Verification items for this drawing (mm, ordinates from the low corner). Coordinates: 2 decimals unless noted, no trailing zeros. Write each loop counter-clockwise with the first axis right and the second up, starting at its lowest first coordinate (ties: lowest second). Pieces come first, ordered by that corner, then holes. Notation, with made-up numbers: M 68.25,60 L 123.25,60 A20 cw 123.25,64 Z; hole C -27.75,51 d3. An arc over 180 degrees is marked long. Answer as CSV lines item,"result". Start each with the question number.
1) Section check B-B (x = 28). Record the cut outline in (y, z) (1 decimal).
2) Section check D-D (z = 11.5). Record the cut outline in (x, y).
3) Material ranges on L1, parallel to X at y = 2.5, z = 41 (1 decimal); L2, parallel to X at y = 3.45, z = 23.5 (1 decimal); L3, parallel to X at y = 1.75, z = 3.5, recorded low to high. Write a range as [from, to].
4) Section check C-C (z = 23.5). Record the cut outline in (x, y).
5) Go/stop test with flat-tipped pins: pin 1 Ø1.7 at (x, z) = (2.8, 42.8) entering from +Y; pin 2 Ø1 at (y, z) = (1, 32) entering from -X (1 decimal); pin 3 Ø3.5 at (x, z) = (37.8, 22.8) entering from +Y; pin 4 Ø2 at (y, z) = (2.5, 8.5) entering from -X. Record where each tip stops, or that it passes through.
6) Draft check along Z on the marked faces 1, 2, 3 and 4. Enter one of: +Z half, -Z half, draft (parallel to the pull), parting line (faces both ways), or undercut.
7) Section check A-A (y = 1.75). State how many separate pieces and enclosed holes the cut face has, and give its area (3 significant figures).
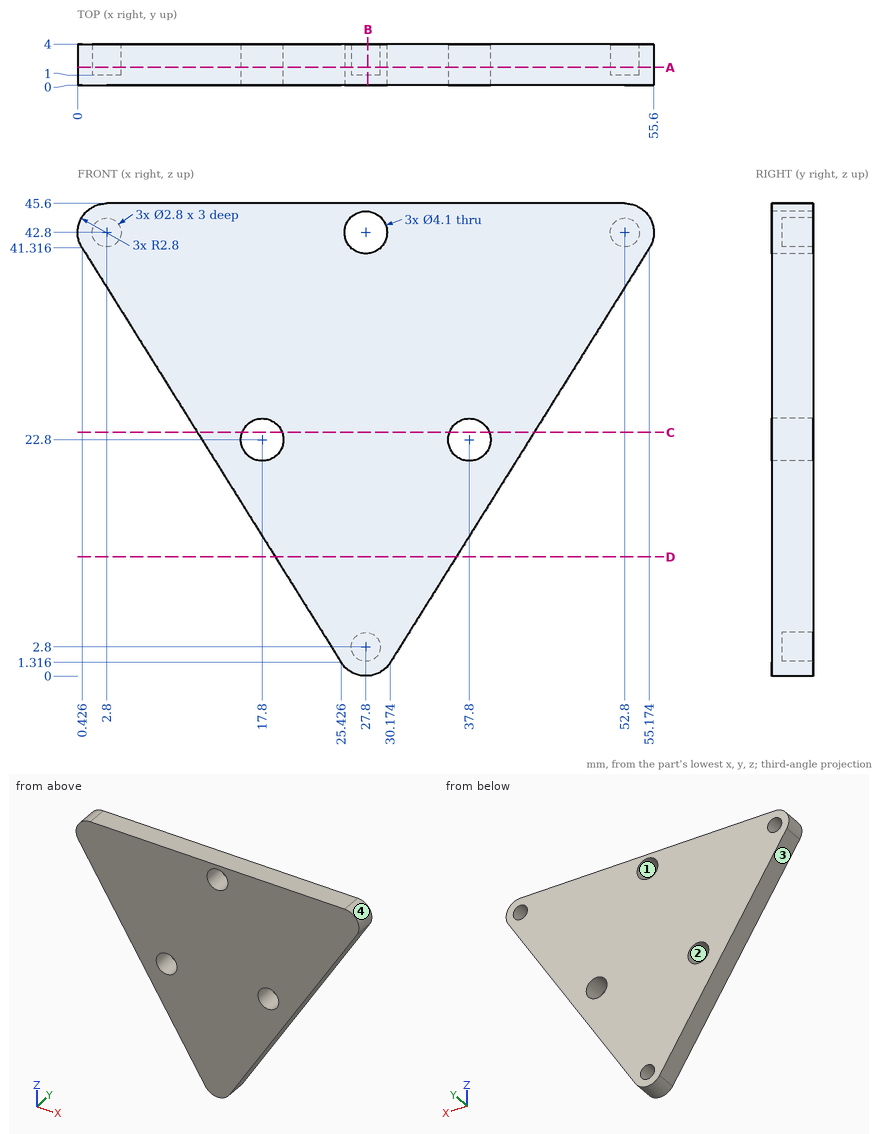
Results found:
1,outline,"M 0,0 L 4,0 L 4,1.4 L 1,1.4 L 1,4.2 L 4,4.2 L 4,40.8 L 0,40.8 Z; M 0,44.8 L 4,44.8 L 4,45.6 L 0,45.6 Z"
2,outline,"M 19.06,0 L 36.54,0 L 36.54,4 L 19.06,4 Z"
3,L1,"x = [0.6, 26.8], [28.8, 55]"
3,L2,"x = [11.6, 15.9], [19.7, 35.9], [39.7, 44]"
3,L3,"x = [24.06, 26.59], [29.01, 31.54]"
4,outline,"M 11.56,0 L 15.87,0 L 15.87,4 L 11.56,4 Z; M 19.73,0 L 35.87,0 L 35.87,4 L 19.73,4 Z; M 39.73,0 L 44.04,0 L 44.04,4 L 39.73,4 Z"
5,pin 1,"stops at y = 1"
5,pin 2,"stops at x = 5.9"
5,pin 3,"passes through"
5,pin 4,"stops at x = 20.31"
6,face 1,"undercut"
6,face 2,"undercut"
6,face 3,"-Z half"
6,face 4,"parting line"
7,separate pieces,"1"
7,enclosed holes,"6"
7,area,"1,370 mm2"
